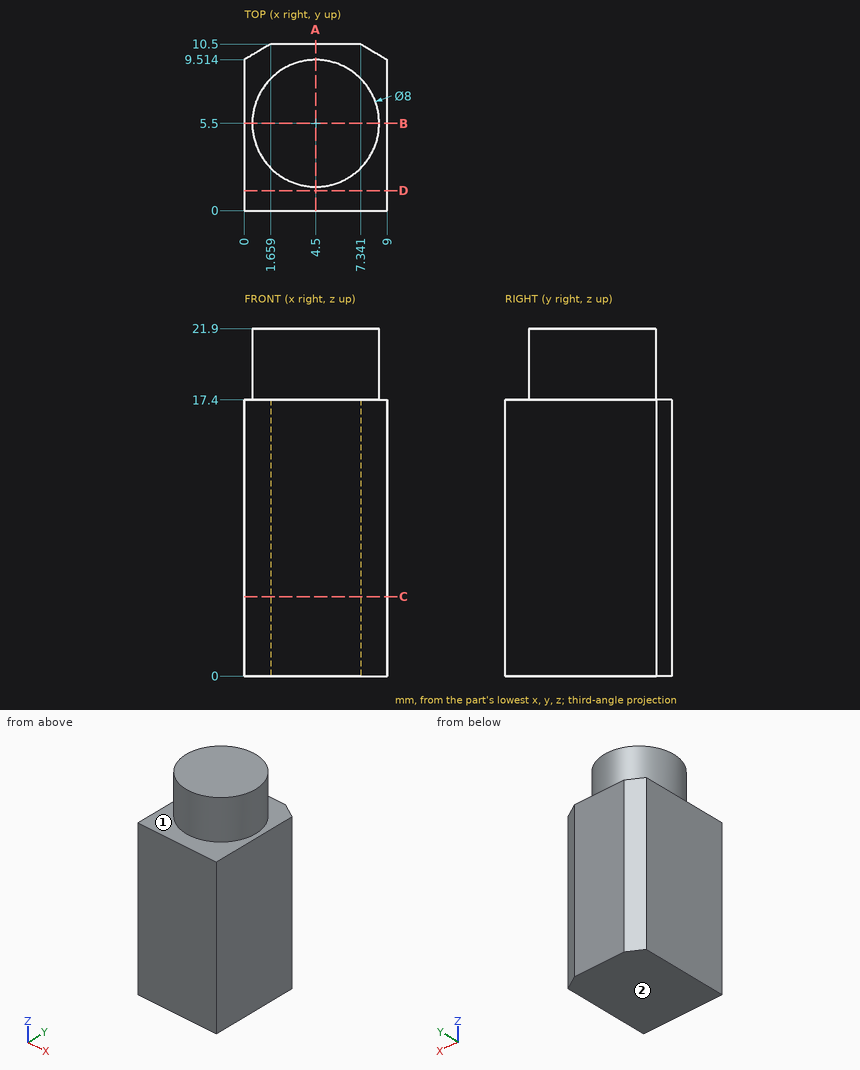
Input: dimensioned drawing with shaded views. Units: mm. Origin: part minimum x, y, z. A direction names the side the tool comes from. Coordinates: 2 decimals unless noted, no trailing zeros. Loops run counter-clockwise (first coordinate to the right, second up) from the corner with the lowest first, then second, coordinate; pieces in that order, holes last. Notation, with made-up numbers: M 66.25,74 L 115.25,74 A36 cw 115.25,109 Z; hole C -11.5,75 d2. An arc over 180 degrees is marked long. One line per item, written item: value.
(1) Section D-D (y = 1.25). Output: boundary loops of the cut face in (x, z), and give its area (3 significant figures).
Filled in:
outline: M 0,0 L 9,0 L 9,17.4 L 0,17.4 Z
area: 157 mm^2
(2) Line query: line 1 along Z through (x, y) = (8, 0.5); line 2 along Y through (x, z) = (1, 15.75); line 3 along Y through (x, z) = (3.5, 19.25). Output: solid intervals per line, ascending. Write a range as from..to.
Filled in:
line 1: 0..17.4
line 2: 0..10.11
line 3: 1.63..9.37
(3) Section A-A (x = 4.5). Output: boundary loops of the cut face in (y, z), and give its area (3 significant figures).
Filled in:
outline: M 0,0 L 10.5,0 L 10.5,17.4 L 9.5,17.4 L 9.5,21.9 L 1.5,21.9 L 1.5,17.4 L 0,17.4 Z
area: 219 mm^2
(4) Reachability of the marked faces 1 and 2 from +Z, -Z, +X, -X, +Y, -Y: full face, straight path, thin tool, end or side. Return the list, or none.
Filled in:
face 1: +Z
face 2: -Z, +X, -X, +Y, -Y
(5) Section B-B (y = 5.5). Output: boundary loops of the cut face in (x, z).
Filled in:
outline: M 0,0 L 9,0 L 9,17.4 L 8.5,17.4 L 8.5,21.9 L 0.5,21.9 L 0.5,17.4 L 0,17.4 Z
(6) Section C-C (z = 5). Output: boundary loops of the cut face in (x, y).
Filled in:
outline: M 0,0 L 9,0 L 9,9.51 L 7.34,10.5 L 1.66,10.5 L 0,9.51 Z
